Read the model definition and answer for the solid it produces. Units are mm, in the model's axes. Give positions to 0.01 mm unless a question says otherwise; leave off trailing zeros. Loops run counter-clockwise (first coordinate to the right, second up) from the corner with the lowest first, then second, coordinate; pieces in that order, holes last.
(1) Determine the mould class of faces 1 (the face through (-17.02, -5.36, 41.6)), 2 (the face through (23, 20, 20.259)), 3 (the face through (-33.494, 13.887, 23.003)) for opening direction X: pulls with the +X half, pulls with the -X half, needs draft (parallel to the pull), parting line crosses it, or undercut.
(2) Find section A-A, the plane z = 37.5. Write down the section's boundary in (x, y), then the cut area to 3 significant figures.
(3) Each of these flat-tipped pins is pushed along its axis until it touches: P1, Ø6, axis at x = 26, y = -3.5, coming from the -Z side; P2, Ø2, axis at x = 28.5, y = 23.5, coming from the -Z side; P3, Ø5, axis at y = -8.5, z = 27, coming from the -X side; P4, Ø3, axis at x = 19, y = -0.5, coming from the +Z side. Where does it stop, or does it pass through?
(4) Find section B-B, the plane z = 26. Write down the section's boundary in (x, y).
(5) Straight lines are drawn through the part: probe 1 along Y at (x, z) = (-20, 22); probe 2 along X at (y, z) = (22, 25); probe 3 along X at (y, z) = (-13, 42.5). For each, find the intervals that lie inside material, in ascending order.
```python
from build123d import *

# Parameters (mm, degrees)
F5_R = 2.5


# Not quite as in the source:
# - the program builds the solid bodies; features that only make, move or delete a surface that nothing else refers to are left out


with BuildPart() as f4:
    # F3 (on Front) → F4 (revolve)
    with BuildSketch(Plane.XZ):
        Polygon((-36.259230652, 20.2593781938), (-28.4696114573, 20.2593781938), (-14.1603897064, 49), (-19.8540338413, 49), (-36.259230652, 24), align=None)
    revolve(axis=Axis((0, 0, 18.828805536), (0, 0, 1)))

    # F5
    f5_edges = [f4.edges().sort_by_distance(p)[0] for p in [
        (19.854034, 0, 49),
        (14.16039, 0, 49),
        (36.259231, 0, 24),
        (36.259231, 0, 20.259378),
        (28.469611, 0, 20.259378),
    ]]
    fillet(f5_edges, radius=F5_R)


solid = f4.part
```
Entries:
1. face 1: undercut
1. face 2: needs draft
1. face 3: parting line crosses it
2. outline: circle Ø54.8 at (0, 0); hole circle Ø39.77 at (0, 0)
2. area: 1,120 mm2
3. P1: stops at z = 20.39
3. P2: stops at z = 21.54
3. P3: stops at x = -35.01
3. P4: stops at z = 49
4. outline: circle Ø69.89 at (0, 0); hole circle Ø51.22 at (0, 0)
5. probe 1: y = -30.1 to -19.02, 19.02 to 30.1
5. probe 2: x = -27.99 to -14.06, 14.06 to 27.99
5. probe 3: x = -20.32 to -11.56, 11.56 to 20.32
